```python
from build123d import *

# Parameters (mm, degrees)
F0_W     = 12.446
F0_H     = 431.8
F0_R     = 3.175
F1_DEPTH = 12.7


with BuildPart() as f1:
    # F0 (on Top) → F1 (new body)
    with BuildSketch(Plane.XY):
        Polygon((602.978926, 205.187889), (-616.221074, 205.187889), (-1022.621074, -99.612111), (-616.221074, -404.412111), (602.978926, -404.412111), align=None)
        with Locations((202.801926, -112.431925)):
            Rectangle(F0_W, F0_H, mode=Mode.SUBTRACT)
        with Locations((-877.206781, -99.612111)):
            Circle(F0_R, mode=Mode.SUBTRACT)
    extrude(amount=F1_DEPTH)


solid = f1.part
```
Model file for the job. Use its own axes, mm. Coordinates: 2 decimals unless noted, no trailing zeros. Write each loop counter-clockwise with the first axis right and the second up, starting at its lowest first coordinate (ties: lowest second). Pieces come first, ordered by that corner, then holes. Notation, with made-up numbers: (13, 5) - (71, 5) arc R26 ccw to (71, 26) - close; hole circle Ø4 at (22, -22.75). An arc over 180 degrees is marked (long way). Use a Markdown table: item, result. Add a question column.
Item 1: Band-saw the part on D-D, the plane y = 153.5. Write the cut outline in (x, z).
Item 2: Band-saw the part on C-C, the plane y = -5.5. Write the cut outline in (x, z), and give its area (3 significant figures).
Item 3: Drill centre lines: line 1 along X through (y, z) = (-40.5, 3); line 2 along X through (y, z) = (-231.5, 3.75); line 3 along Y through (x, z) = (-804, 1.25). Where is each one in solid material? Low to high.
Item 4: Drop flat-ended pins along their axis: pin 1 (2 mm diameter, centred on x = -706, z = 8.5, fed in from +Y); pin 2 (3 mm diameter, centred on x = -653.5, z = 4, fed in from -Y); pin 3 (4 mm diameter, centred on y = -161, z = 8, fed in from -X). Give the stop position or say it passes through.
Item 5: Band-saw the part on A-A, the plane z = 3.75. Write the cut outline in (x, y) (3 decimals).
Item 6: Band-saw the part on B-B, the plane y = -228. Write the cut outline in (x, z), and give its area (3 significant figures).
A:
| question | item | result |
|---|---|---|
| 1 | outline | (-685.14, 0) - (602.98, 0) - (602.98, 12.7) - (-685.14, 12.7) - close |
| 2 | outline | (-897.14, 0) - (196.58, 0) - (196.58, 12.7) - (-897.14, 12.7) - close; (209.02, 0) - (602.98, 0) - (602.98, 12.7) - (209.02, 12.7) - close |
| 2 | area | 18,900 mm² |
| 3 | line 1 | x = -943.8 to 196.58, 209.02 to 602.98 |
| 3 | line 2 | x = -846.77 to 196.58, 209.02 to 602.98 |
| 3 | line 3 | y = -263.58 to 64.35 |
| 4 | pin 1 | stops at y = 138.6 |
| 4 | pin 2 | stops at y = -377.58 |
| 4 | pin 3 | stops at x = -943.44 |
| 5 | outline | (-1022.621, -99.612) - (-616.221, -404.412) - (602.979, -404.412) - (602.979, 205.188) - (-616.221, 205.188) - close; hole circle Ø6.35 at (-877.207, -99.612); hole (196.579, -328.332) - (209.025, -328.332) - (209.025, 103.468) - (196.579, 103.468) - close |
| 6 | outline | (-851.44, 0) - (196.58, 0) - (196.58, 12.7) - (-851.44, 12.7) - close; (209.02, 0) - (602.98, 0) - (602.98, 12.7) - (209.02, 12.7) - close |
| 6 | area | 18,300 mm² |
